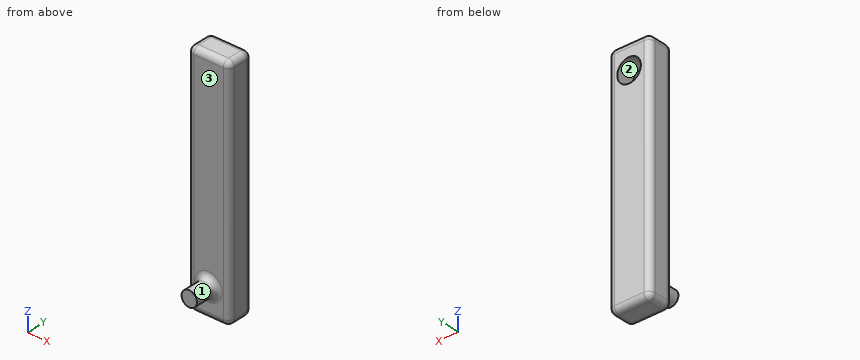
from build123d import *

# Parameters (mm, degrees)
F0_W     = 3.5
F0_H     = 20
F1_DEPTH = 2.2
F2_R     = 1
F3_DEPTH = 1.5
F4_R     = 0.65
F5_DEPTH = 1.9
F6_R     = 0.5


with BuildPart() as f1:
    # F0 (on Front) → F1 (new body)
    with BuildSketch(Plane.XZ):
        Rectangle(F0_W, F0_H)
    extrude(amount=F1_DEPTH)

    # F2 (on face) → F3 (cut)
    with BuildSketch(Plane(origin=(0, 0, 0), x_dir=(-1, 0, 0), z_dir=(0, 1, 0))):
        with Locations((0, 7.771334)):
            Circle(F2_R)
    extrude(amount=-F3_DEPTH, mode=Mode.SUBTRACT)

    # F4 (on face) → F5 (join)
    with BuildSketch(Plane.XZ.offset(2.2)):
        with Locations((0, -7.556978)):
            Circle(F4_R)
    extrude(amount=F5_DEPTH)

    # F6
    f6_edges = [f1.edges().sort_by_distance(p)[0] for p in [
        (1.75, -1.1, -10),
        (1.75, -1.1, 10),
        (1.75, 0, 0),
        (1.75, -2.2, 0),
        (0, -2.2, -10),
        (-1.75, -2.2, 0),
        (0, -2.2, 10),
        (-0.65, -2.2, -7.556978),
        (-1.75, -1.1, 10),
        (-1.75, -1.1, -10),
        (-1.75, 0, 0),
        (0, 0, 10),
        (0, 0, -10),
    ]]
    fillet(f6_edges, radius=F6_R)


solid = f1.part
Verification items for the finished model (mm, model axes). Face numbers are marked on the shaded views. Coordinates: 2 decimals unless noted, no trailing zeros. Loops run counter-clockwise (first coordinate to the right, second up) from the corner with the lowest first, then second, coordinate; pieces in that order, holes last. Notation, with made-up numbers: M -7,17.5 L 14,17.5 A38 cw 14,55.5 Z; hole C -6.5,29.25 d6. An arc over 180 degrees is marked long. One line per item, written item: value.
1. Gauge pin test, flat ends, axial feed: P1, Ø1.5, axis at y = -2.5, z = -2, coming from the -X side; P2, Ø1, axis at x = 0.5, y = -2.5, coming from the +Z side; P3, Ø0.8, axis at x = 0.5, z = 4, coming from the -Y side. Record the tip position at first contact, or that the pin passes through.
Answers follow:
P1: x = -1.75
P2: z = 9.9
P3: y = -2.2
2. Section check A-A on x = 0. Record the cut outline in (y, z).
Answers follow:
outline: M -4.1,-8.21 L -2.7,-8.21 A0.5 cw -2.2,-8.71 L -2.2,-9.5 A0.5 ccw -1.7,-10 L -0.5,-10 A0.5 ccw 0,-9.5 L 0,6.77 L -1.5,6.77 L -1.5,8.77 L 0,8.77 L 0,9.5 A0.5 ccw -0.5,10 L -1.7,10 A0.5 ccw -2.2,9.5 L -2.2,-6.41 A0.5 cw -2.7,-6.91 L -4.1,-6.91 Z
3. Mould release check, pull along Z, two halves, no side actions. Record for the marked faces 1, 2 and 3: pulls with the +Z half, pulls with the -Z half, needs draft (parallel to the pull), parting line crosses it, or undercut.
Answers follow:
face 1: parting line crosses it
face 2: undercut
face 3: needs draft
4. Section check C-C on y = -3.5. Record the cut outline in (x, z).
Answers follow:
outline: C 0,-7.56 d1.3
5. Material ranges on line 1 along Z through (x, y) = (0, -1.2); line 2 along Y through (x, z) = (-0.5, -3.5); line 3 along Y through (x, z) = (0.35, 8.25), recorded low to high. Write a range as from..to.
Answers follow:
line 1: -10..6.77, 8.77..10
line 2: -2.2..0
line 3: -2.2..-1.5
6. Section check B-B on z = 3.5. Record the cut outline in (x, y).
Answers follow:
outline: M -1.75,-1.7 A0.5 ccw -1.25,-2.2 L 1.25,-2.2 A0.5 ccw 1.75,-1.7 L 1.75,-0.5 A0.5 ccw 1.25,0 L -1.25,0 A0.5 ccw -1.75,-0.5 Z
